Geometry: see drawing. Coordinates: mm, zero at the bounding-box minimum. A direction names the side the tool comes from. Coordinates: 2 decimals unless noted, no trailing zeros. Order: outer loops, then holes, each group sorted by start corner. A loop starts at its lowest first (then second) coordinate and runs counter-clockwise, first axis right, second up. Notation, with made-up numbers: M 42.5,36 L 92.5,36 A14 ccw 92.5,60 Z; hole C 82,30 d8. An arc over 180 degrees is marked long. Answer in a Markdown table with one row per item.
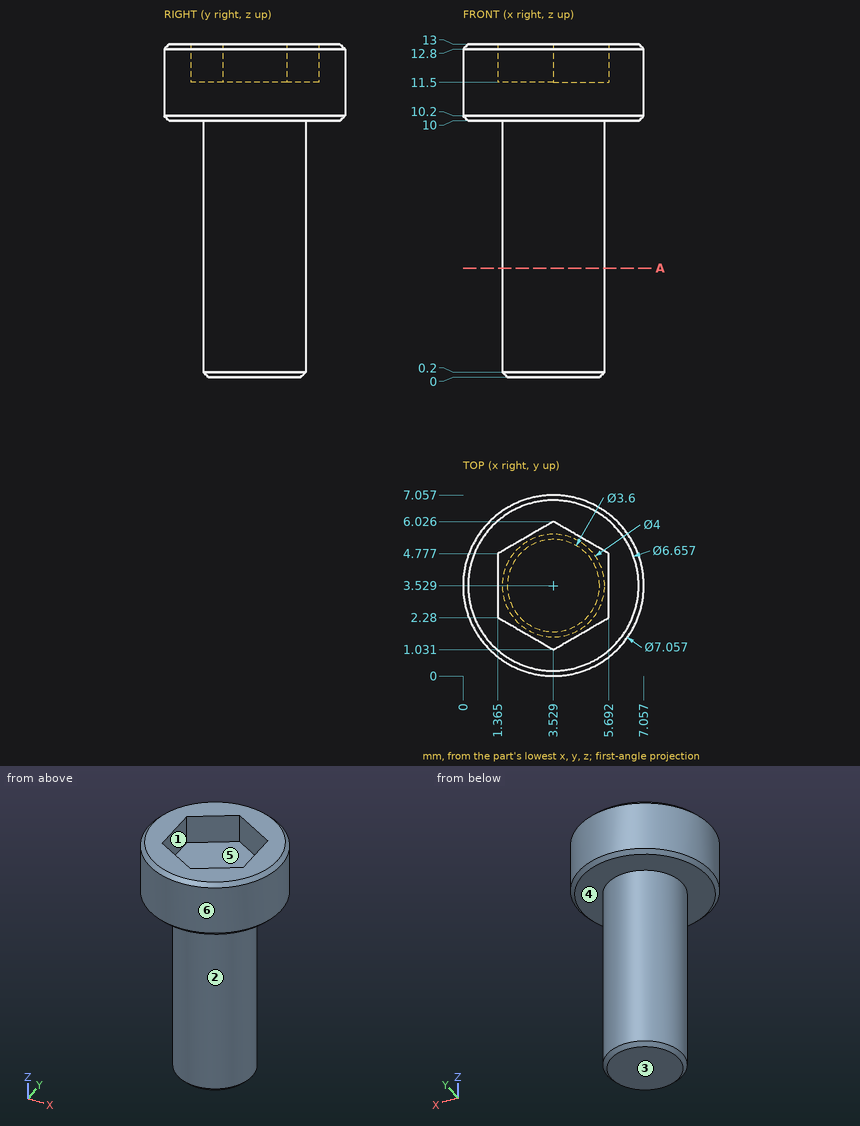
1) Reachability of the marked faces 1, 2 and 3 from +Z, -Z, +X, -X, +Y, -Y: full face, straight path, thin tool, end or side. Return the list, or none.
Resolved:
| item | result |
|---|---|
| face 1 | +Z |
| face 2 | -Z |
| face 3 | -Z, +X, -X, +Y, -Y |
2) Mould query, pull axis Y, two halves, no side actions, for the marked faces 4, 5 and 6. Classes: +Y half, -Y half, draft (parallel to the pull), parting line (faces both ways), or undercut.
Resolved:
| item | result |
|---|---|
| face 4 | draft |
| face 5 | undercut |
| face 6 | parting line |
3) Cut plane A-A, the plane z = 4.25. Output: boundary loops of the cut face in (x, y), and give its area (3 significant figures).
Resolved:
| item | result |
|---|---|
| outline | C 3.53,3.53 d4 |
| area | 12.6 mm2 |
4) Contact query for flat-ended pins moving along their axis: pin 1 (1 mm diameter, centred on y = 6, z = 11, fed in from -X); pin 2 (2 mm diameter, centred on x = 3.5, y = 3.5, fed in from +Z); pin 3 (1.2 mm diameter, centred on y = 3, z = 12, fed in from -X); pin 4 (4 mm diameter, centred on x = 3.5, z = 1.5, fed in from -Y). Output: stop coordinate, or through.
Resolved:
| item | result |
|---|---|
| pin 1 | stops at x = 0.6 |
| pin 2 | stops at z = 11.5 |
| pin 3 | stops at x = 0 |
| pin 4 | stops at y = 1.53 |
5) Material intervals for probe 1 along Z at (x, y) = (4.75, 5.5); probe 2 along Z at (x, y) = (4, 2.5); probe 3 along Y at (x, z) = (3, 5.75), sorted ascending.
Resolved:
| item | result |
|---|---|
| probe 1 | z = 10 to 13 |
| probe 2 | z = 0 to 11.5 |
| probe 3 | y = 1.6 to 5.46 |
